Read the model definition and answer for the solid it produces. Units are mm, in the model's axes. A direction names the side the tool comes from. Give positions to 0.01 mm unless a question says otherwise; leave off trailing zeros. Order: outer loops, then holes, each group sorted by start corner. A loop starts at its lowest first (then second) coordinate and runs counter-clockwise, first axis right, second up. Notation, with made-up numbers: (49, -4.5) -> (59, -4.5) arc R16 ccw to (59, 20.5) -> close; hole circle Ø7 at (21.25, 7). An arc over 180 degrees is marked (long way). Use one line per item in the form item = value.
```python
from build123d import *

# Parameters (mm, degrees)
F3_DEPTH  = 0.4
F4_DEPTH  = 0.65
F5_ANGLE  = 90
F9_ANGLE  = -90
F11_ANGLE = 180
F13_DEPTH = 0.6
F14_R     = 0.1675
F17_DEPTH = 0.1


# Not quite as in the source:
# - a feature of the source that left no trace in its solid (it failed there, or was rolled back) is left out


with BuildPart() as f3:
    # F2 (on Front) → F3 (new body)
    with BuildSketch(Plane.XZ):
        with BuildLine():
            Line((0, 0.3), (0, 0))
            Line((0, 0), (3.6876645899, 0))
            ThreePointArc((3.6876645899, 0), (3.7184315179, 0.004850664), (3.7462136453, 0.0189320772))
            Line((3.7462136453, 0.0189320772), (3.9709811077, 0.1812641333))
            ThreePointArc((3.9709811077, 0.1812641333), (4.5807248826, 0.8921178442), (4.8, 1.8026225901))
            Line((4.8, 1.8026225901), (4.8, 3.5100976163))
            ThreePointArc((4.8, 3.5100976163), (4.6627693477, 4.1368828306), (4.2761870602, 4.6489825198))
            Line((4.2761870602, 4.6489825198), (2.8404336486, 5.8796283012))
            ThreePointArc((2.8404336486, 5.8796283012), (2.6885110858, 5.9689425075), (2.5150379619, 6))
            Line((2.5150379619, 6), (0, 6))
            Line((0, 6), (0, 5.55))
            Line((0, 5.55), (2.5733712952, 5.55))
            ThreePointArc((2.5733712952, 5.55), (2.60806592, 5.5437885015), (2.6384504326, 5.5259256602))
            Line((2.6384504326, 5.5259256602), (4.0158705108, 4.3452798789))
            ThreePointArc((4.0158705108, 4.3452798789), (4.2993641883, 3.9697401068), (4.4, 3.5100976163))
            Line((4.4, 3.5100976163), (4.4, 1.812848816))
            ThreePointArc((4.4, 1.812848816), (4.2223871549, 1.0753399719), (3.7284946972, 0.499548466))
            Line((3.7284946972, 0.499548466), (3.4521968212, 0.3))
            Line((3.4521968212, 0.3), (0, 0.3))
        make_face()
    extrude(amount=F3_DEPTH)

    # F4 (add): a face of the model
    f4_faces = [f3.faces().sort_by_distance(p)[0] for p in [
        (0, -0.2, 5.775),
    ]]
    extrude(f4_faces, amount=F4_DEPTH)

    # F2 (on Front) → F5 (revolve)
    with BuildSketch(Plane.XZ):
        with BuildLine():
            Line((0, 0.3), (0, 0))
            Line((0, 0), (3.6876645899, 0))
            ThreePointArc((3.6876645899, 0), (3.7184315179, 0.004850664), (3.7462136453, 0.0189320772))
            Line((3.7462136453, 0.0189320772), (3.9709811077, 0.1812641333))
            ThreePointArc((3.9709811077, 0.1812641333), (4.5807248826, 0.8921178442), (4.8, 1.8026225901))
            Line((4.8, 1.8026225901), (4.8, 3.5100976163))
            ThreePointArc((4.8, 3.5100976163), (4.6627693477, 4.1368828306), (4.2761870602, 4.6489825198))
            Line((4.2761870602, 4.6489825198), (2.8404336486, 5.8796283012))
            ThreePointArc((2.8404336486, 5.8796283012), (2.6885110858, 5.9689425075), (2.5150379619, 6))
            Line((2.5150379619, 6), (0, 6))
            Line((0, 6), (0, 5.55))
            Line((0, 5.55), (2.5733712952, 5.55))
            ThreePointArc((2.5733712952, 5.55), (2.60806592, 5.5437885015), (2.6384504326, 5.5259256602))
            Line((2.6384504326, 5.5259256602), (4.0158705108, 4.3452798789))
            ThreePointArc((4.0158705108, 4.3452798789), (4.2993641883, 3.9697401068), (4.4, 3.5100976163))
            Line((4.4, 3.5100976163), (4.4, 1.812848816))
            ThreePointArc((4.4, 1.812848816), (4.2223871549, 1.0753399719), (3.7284946972, 0.499548466))
            Line((3.7284946972, 0.499548466), (3.4521968212, 0.3))
            Line((3.4521968212, 0.3), (0, 0.3))
        make_face()
    revolve(axis=Axis((0, 0, 5.775), (0, 0, 1)), revolution_arc=F5_ANGLE)


with BuildPart() as f9_1:
    # F9: copy of F3
    add(f3.part.rotate(Axis((-0.2, -0.2, 0.1248804607), (0, 0, 1)), F9_ANGLE))


with BuildPart() as f3_1:
    add(f3.part)

    # F10: union F9_1
    add(f9_1.part)


with BuildPart() as f11_1:
    # F11: copy of F3
    add(f3_1.part.rotate(Axis((-0.2, -0.2, 0.1248804607), (0, 0, 1)), F11_ANGLE))


with BuildPart() as f3_2:
    add(f3_1.part)

    # F12: union F11_1
    add(f11_1.part)

    # F13 (add): a face of the model
    f13_faces = [f3_2.faces().sort_by_distance(p)[0] for p in [
        (-0.2, 0, 0.15),
    ]]
    extrude(f13_faces, amount=F13_DEPTH)

    # F14 (on face) → F17 (join)
    with BuildSketch(Plane(origin=(0, 0, 0), x_dir=(1, 0, 0), z_dir=(0, 0, -1))):
        Circle(F14_R)
    extrude(amount=F17_DEPTH)


solid = f3_2.part
```
Item 1: Which of the six approach directions +Z, -Z, +X, -X, +Y, -Y give full straight-line access (tool end or side, diameter ignored) to faces 1 (the flat face through (0, 0, 6)), 2 (the cylindrical face through (-3.477, 3.145, 2.65))?
Checks:
face_1 = +Z, +X, -X, +Y, -Y
face_2 = none
Item 2: The part is cut by section A-A on z = 3.25. Give the vertices of the cut face in (x, y), and give its area (3 significant figures).
Checks:
outline = (-5.2, -0.4) arc R4.8 ccw to (-0.4, -5.2) -> (0, -5.2) arc R4.8 ccw to (4.8, -0.4) -> (4.8, 0) arc R4.8 ccw to (0, 4.8) -> (-0.4, 4.8) arc R4.8 ccw to (-5.2, 0) -> close; hole (-4.8, -0.4) arc R4.4 ccw to (-0.4, -4.8) -> (0, -4.8) arc R4.4 ccw to (4.4, -0.4) -> (4.4, 0) arc R4.4 ccw to (0, 4.4) -> (-0.4, 4.4) arc R4.4 ccw to (-4.8, 0) -> close
area = 12.2 mm²
Item 3: Given pin 1 Ø1 at (x, z) = (1.5, 4) entering from -Y; pin 2 Ø1 at (y, z) = (-3.5, 4.5) entering from +X; pin 3 Ø4 at (x, y) = (-4, -3) entering from -Z; pin 4 Ø6 at (x, y) = (-2, 1.5) entering from -Z, each flat-ended and moving along its own axis, determine where each tip first touches the part or whether it passes through.
Checks:
pin_1 = -5.06
pin_2 = 3.76
pin_3 = 0
pin_4 = -0.1
Item 4: The part is cut by section B-B on z = 5.25. Give the vertices of the cut face in (x, y) (3 decimals).
Checks:
outline = (-3.975, -0.4) arc R3.575 ccw to (-0.4, -3.975) -> (0, -3.975) arc R3.575 ccw to (3.575, -0.4) -> (3.575, 0) arc R3.575 ccw to (0, 3.575) -> (-0.4, 3.575) arc R3.575 ccw to (-3.975, 0) -> close; hole (-3.36, -0.4) arc R2.96 ccw to (-0.4, -3.36) -> (0, -3.36) arc R2.96 ccw to (2.96, -0.4) -> (2.96, 0) arc R2.96 ccw to (0, 2.96) -> (-0.4, 2.96) arc R2.96 ccw to (-3.36, 0) -> close
Item 5: Straight lines are drawn through the part: L1, parallel to Z at x = 0.5, y = 1.25; L2, parallel to X at y = -2.5, z = 4.5; L3, parallel to X at y = 1.25, z = 4. For each, find the intervals that lie inside material, in ascending order. Write a range as from..to.
Checks:
L1 = 0..0.3, 5.55..6
L2 = -4.3..-3.61, 3.21..3.9
L3 = -4.95..-4.5, 4.1..4.55
Item 6: Determine the mould class of faces 3 (the cylindrical face through (-3.83, -3.76, 2.67)), 4 (the flat face through (0, 0, 5.55)), 5 (the flat face through (-0.203, 3.568, 5.256)) for opening direction X: +X half, -X half, draft (parallel to the pull), parting line (faces both ways), or undercut.
Checks:
face_3 = -X half
face_4 = undercut
face_5 = draft
